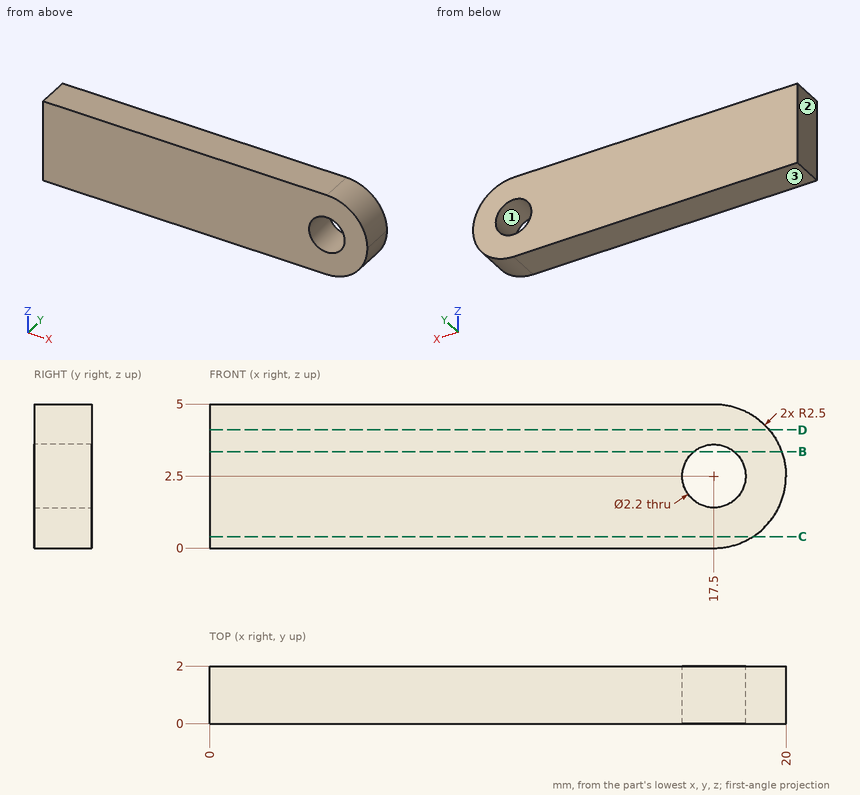
The figure shows three views and two pictorial views of one solid part (mm, origin at its lowest corner). Answer the questions. Give positions to 0.01 mm unless a question says otherwise; leave off trailing zeros. Loops run counter-clockwise (first coordinate to the right, second up) from the corner with the lowest first, then second, coordinate; pieces in that order, holes last. Notation, with made-up numbers: (15.5, 46.25) -> (21.5, 46.25) arc R30 cw to (21.5, 80.25) -> close; hole circle Ø8 at (-21.5, 85). An arc over 180 degrees is marked (long way). Put each result on its own line as item: value. Start each with the question number.
Item 1: Find the intervals of material crossed by L1, parallel to X at y = 0.65, z = 2.5; L2, parallel to X at y = 0.6, z = 1.6; L3, parallel to Z at x = 17.25, y = 1.1, in increasing order. Write a range as [from, to].
Item 2: The part is cut by section D-D (z = 4.1). Give the vertices of the cut face in (x, y).
Item 3: The part is cut by section B-B (z = 3.35). Give the vertices of the cut face in (x, y).
Item 4: The part is cut by section C-C (z = 0.4). Give the vertices of the cut face in (x, y).
Item 5: The mould has two halves that part along X. Classify the marked faces 1, 2 and 3: released by +X, released by -X, zero draft, split by the parting line, or undercut.
Item 6: This flat-tipped pin is pushed along its axis until it touches: P1, Ø2, axis at x = 17.5, z = 2.5, coming from the -Y side. Where does it stop, or does it pass through?
Answers below:
1. L1: [0, 16.4], [18.6, 20]
1. L2: [0, 16.87], [18.13, 19.83]
1. L3: [0, 1.43], [3.57, 5]
2. outline: (0, 0) -> (19.42, 0) -> (19.42, 2) -> (0, 2) -> close
3. outline: (0, 0) -> (16.8, 0) -> (16.8, 2) -> (0, 2) -> close; (18.2, 0) -> (19.85, 0) -> (19.85, 2) -> (18.2, 2) -> close
4. outline: (0, 0) -> (18.86, 0) -> (18.86, 2) -> (0, 2) -> close
5. face 1: undercut
5. face 2: released by -X
5. face 3: zero draft
6. P1: through
